Work out the finished part from the listing and answer in its coordinate system (mm). Face numbers are marked on the shaded views. A direction names the side the tool comes from. Coordinates: 2 decimals unless noted, no trailing zeros. Write each loop counter-clockwise with the first axis right and the second up, starting at its lowest first coordinate (ties: lowest second). Pieces come first, ordered by that corner, then holes. Notation, with made-up numbers: (62, 85.5) - (72, 85.5) arc R9 cw to (72, 98.5) - close; hole circle Ø7 at (84.5, -17). An arc over 180 degrees is marked (long way). One line per item, written item: value.
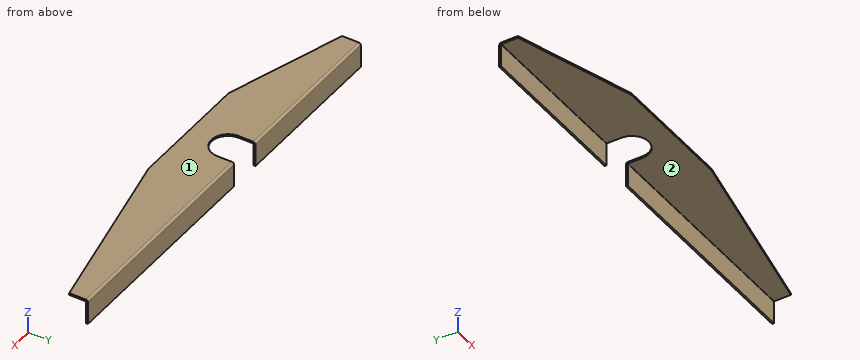
```python
from build123d import *

# Parameters (mm, degrees)
BASE_FLANGE1_DEPTH             = 1.5
EDGE_FLANGE1_STRIP_W           = 6.4
EDGE_FLANGE1_STRIP_H           = 1.5
EDGE_FLANGE1_STRIP_CUT_DEPTH   = 131.65
EDGE_FLANGE1_STRIP_2_W         = 6.4
EDGE_FLANGE1_STRIP_2_H         = 1.5
EDGE_FLANGE1_STRIP_CUT_2_DEPTH = 182.65
EDGE_FLANGE1_DEPTH             = 131.65
EDGE_FLANGE1_BEND_DEPTH        = 182.65


# Sheet-metal steps are written as plain solids
with BuildPart() as part:
    # Sketch1 → Base-Flange1 (new body)
    with BuildSketch(Plane.XY):
        with BuildLine():
            Line((13.35, 0), (13.35, 13.35))
            Line((13.35, 13.35), (196, 13.35))
            Line((196, 13.35), (196, -1.65))
            Line((196, -1.65), (50, -31.65))
            Line((50, -31.65), (-50, -31.65))
            Line((-50, -31.65), (-145, -1.65))
            Line((-145, -1.65), (-145, 13.35))
            Line((-145, 13.35), (-13.35, 13.35))
            Line((-13.35, 13.35), (-13.35, 0))
            ThreePointArc((-13.35, 0), (0, -13.35), (13.35, 0))
        make_face()
    extrude(amount=-BASE_FLANGE1_DEPTH)

    # Edge-Flange1 strip (across the edge) → Edge-Flange1 strip cut (cut)
    with BuildSketch(Plane(origin=(-145, 13.35, -1.5), x_dir=(0, -1, 0), z_dir=(1, 0, 0))):
        with Locations((-1.5, -0.75)):
            Rectangle(EDGE_FLANGE1_STRIP_W, EDGE_FLANGE1_STRIP_H)
    extrude(amount=EDGE_FLANGE1_STRIP_CUT_DEPTH, mode=Mode.SUBTRACT)

    # Edge-Flange1 strip 2 (across the edge) → Edge-Flange1 strip cut 2 (cut)
    with BuildSketch(Plane(origin=(13.35, 13.35, -1.5), x_dir=(0, -1, 0), z_dir=(1, 0, 0))):
        with Locations((-1.5, -0.75)):
            Rectangle(EDGE_FLANGE1_STRIP_2_W, EDGE_FLANGE1_STRIP_2_H)
    extrude(amount=EDGE_FLANGE1_STRIP_CUT_2_DEPTH, mode=Mode.SUBTRACT)

    # Edge-Flange1 section (across the edge) → Edge-Flange1 (add)
    with BuildSketch(Plane(origin=(-145, 13.35, -1.5), x_dir=(0, -1, 0), z_dir=(1, 0, 0))):
        with BuildLine():
            Line((0, 0.2), (0, 18.5))
            Line((0, 18.5), (1.5, 18.5))
            Line((1.5, 18.5), (1.5, 0.2))
            ThreePointArc((1.5, 0.2), (1.558578644, 0.058578644), (1.7, 0))
            Line((1.7, 0), (1.7, -1.5))
            ThreePointArc((1.7, -1.5), (0.497918472, -1.002081528), (0, 0.2))
        make_face()
    extrude(amount=EDGE_FLANGE1_DEPTH)

    # Edge-Flange1 section 2 (across the edge) → Edge-Flange1 bend (add)
    with BuildSketch(Plane(origin=(13.35, 13.35, -1.5), x_dir=(0, -1, 0), z_dir=(1, 0, 0))):
        with BuildLine():
            Line((0, 0.2), (0, 18.5))
            Line((0, 18.5), (1.5, 18.5))
            Line((1.5, 18.5), (1.5, 0.2))
            ThreePointArc((1.5, 0.2), (1.558578644, 0.058578644), (1.7, 0))
            Line((1.7, 0), (1.7, -1.5))
            ThreePointArc((1.7, -1.5), (0.497918472, -1.002081528), (0, 0.2))
        make_face()
    extrude(amount=EDGE_FLANGE1_BEND_DEPTH)


solid = part.part
```
Item 1: Section C-C, the plane x = 29.5 is taken. Determine the outline of the cut face in (y, z).
Evaluation:
outline: (-31.65, -1.5) - (11.65, -1.5) arc R0.2 cw to (11.85, -1.7) - (11.85, -20) - (13.35, -20) - (13.35, -1.7) arc R1.7 ccw to (11.65, 0) - (-31.65, 0) - close
Item 2: Given pin 1 (13 mm diameter, centred on x = -1, y = -8, fed in from -Z); pin 2 (4 mm diameter, centred on x = 84, z = -11, fed in from -Y); pin 3 (5 mm diameter, centred on y = -14.5, z = -6, fed in from +X), each flat-ended and moving along its own axis, determine where each tip first touches the part or whether it passes through.
Evaluation:
pin 1: stops at z = -1.5
pin 2: stops at y = 11.85
pin 3: passes through
Item 3: Section B-B, the plane y = -6 is taken. Determine the outline of the cut face in (x, z) (3 decimals), then the cut area to 3 significant figures.
Evaluation:
outline: (-131.225, -1.5) - (-11.926, -1.5) - (-11.926, 0) - (-131.225, 0) - close; (11.926, -1.5) - (174.83, -1.5) - (174.83, 0) - (11.926, 0) - close
area: 423 mm2
Item 4: Consider probe 1 along Y at (x, z) = (147.5, -18.25); probe 2 along Z at (x, y) = (44, 3). Determine where each line is inside the solid, lowest interval first.
Evaluation:
probe 1: y = 11.85 to 13.35
probe 2: z = -1.5 to 0
Item 5: Section D-D, the plane x = -67.5 is taken. Determine the outline of the cut face in (y, z).
Evaluation:
outline: (-26.12, -1.5) - (11.65, -1.5) arc R0.2 cw to (11.85, -1.7) - (11.85, -20) - (13.35, -20) - (13.35, -1.7) arc R1.7 ccw to (11.65, 0) - (-26.12, 0) - close
Item 6: Which of the six approach directions +Z, -Z, +X, -X, +Y, -Y give full straight-line access (tool end or side, diameter ignored) to the marked faces 1 and 2?
Evaluation:
face 1: +Z, +X, -X, +Y, -Y
face 2: -Z, +X, -X, -Y
Item 7: Section A-A, the plane z = -7 is taken. Determine the outline of the cut face in (x, y).
Evaluation:
outline: (-145, 11.85) - (-13.35, 11.85) - (-13.35, 13.35) - (-145, 13.35) - close; (13.35, 11.85) - (196, 11.85) - (196, 13.35) - (13.35, 13.35) - close
